Autodesk Inventor part; units mm, degrees
ref_plane "YZ Plane" through (0, 0, 0) normal (1, 0, 0) x (0, 1, 0)
ref_plane "XZ Plane" through (0, 0, 0) normal (0, 1, 0) x (-1, 0, 0)
ref_plane "XY Plane" through (0, 0, 0) normal (0, 0, 1) x (1, 0, 0)
sketch "Sketch1" plane through (0, 0, 0) normal (0, 1, 0) x (-1, 0, 0)
  line L0 (0, 0) -> (-50, 0)
  line L1 (-50, 0) -> (-50, -50)
  line L2 (-50, -50) -> (0, -50)
  line L3 (0, -50) -> (0, 0)
  line L4 (-5, -5) -> (-45, -5)
  line L5 (-45, -5) -> (-45, -45)
  line L6 (-45, -45) -> (-5, -45)
  line L7 (-5, -45) -> (-5, -5)
  dimension "d0" = 50
  dimension "d1" = 50
  dimension "d2" = 5
extrude "Extrusion1" add sketch "Sketch1" along normal blind 5
sketch "Sketch2" plane through (0, 0, 0) normal (0, 0, 1) x (1, 0, 0)
  line L0 (0, 5) -> (50, 5)
  line L1 (13, 5) -> (37, 5)
  line L2 (37, 5) -> (37, 2.5)
  line L3 (37, 2.5) -> (13, 2.5)
  line L4 (13, 2.5) -> (13, 5)
  line L5 (0, 0) -> (50, 0)
  line L6 (0, 0) -> (0, 5)
  dimension "d5" = 24
  dimension "d6" = 2.5
  dimension "d7" = 13
extrude "Extrusion2" cut sketch "Sketch2" against normal through all
sketch "Sketch3" plane through (0, 0, 0) normal (0, 0, 1) x (1, 0, 0)
  line L0 (13, 2.5) -> (13, 5)
  line L1 (13, 5) -> (13, 15)
  line L2 (13, 5) -> (0, 5)
  line L3 (13, 15) -> (0, 5)
  line L4 (37, 5) -> (37, 2.5)
  line L5 (37, 5) -> (37, 15)
  line L6 (50, 5) -> (37, 5)
  line L7 (37, 15) -> (50, 5)
  point P0 (0, 0)
  dimension "d10" = 10
  dimension "d11" = 10
extrude "Extrusion3" add sketch "Sketch3" against normal blind 5
sketch "Sketch4" plane through (50, 0, -50) normal (0, 0, -1) x (-1, 0, 0)
  line L0 (50, 5) -> (37, 15)
  line L1 (37, 15) -> (37, 2.5)
  line L2 (13, 15) -> (0, 5)
  line L3 (13, 2.5) -> (13, 15)
  line L4 (0, 5) -> (13, 15)
  line L5 (13, 5) -> (5, 5)
  line L6 (13, 15) -> (13, 5)
  line L7 (0, 5) -> (13, 5)
  line L8 (13, 5) -> (0, 5)
  line L9 (50, 5) -> (45, 5)
  line L10 (50, 5) -> (37, 15)
  line L11 (45, 5) -> (37, 5)
  line L12 (37, 15) -> (37, 5)
  line L13 (37, 5) -> (50, 5)
  point P0 (50, 0)
extrude "Extrusion4" add sketch "Sketch4" against normal blind 5
sketch "Sketch5" plane through (50, 0, -50) normal (0, 0, -1) x (-1, 0, 0)
  circle A0 centre (39.5, 9) radius 0.5
  circle A1 centre (10.5, 9) radius 0.5
  line L0 (37, 2.5) -> (13, 2.5)
  line L1 (37, 15) -> (37, 2.5)
  line L2 (13, 2.5) -> (13, 15)
  point P0 (50, 0)
  dimension "d16" = 6.5
  dimension "d17" = 6.5
  dimension "d18" = 1
  dimension "d19" = 1
  dimension "d20" = 2.5
  dimension "d21" = 2.5
sketch "Sketch6" plane through (50, 0, -50) normal (0, 0, -1) x (-1, 0, 0)
  point P0 (50, 0)
extrude "Extrusion5" cut sketch "Sketch5" against normal through all
properties part number "MotorMountForPrograming"
Work out the finished part from the listing and answer in its coordinate system (mm). A direction names the side the tool comes from. Give positions to 0.01 mm unless a question says otherwise; leave off trailing zeros. Write each loop counter-clockwise with the first axis right and the second up, starting at its lowest first coordinate (ties: lowest second). Pieces come first, ordered by that corner, then holes. Notation, with made-up numbers: M 67,-37.75 L 76,-37.75 A16 ccw 76,-22.75 Z; hole C 73.25,48 d5. An arc over 180 degrees is marked long. Answer as CSV lines item,"result".
Q1. Find the intervals of material crossed by probe 1 along X at (y, z) = (5, -4); probe 2 along Z at (x, y) = (7, 2.25); probe 3 along Y at (x, z) = (19, -3.5), in increasing order. Write a range as [from, to].
A:
probe 1,"x = [0, 13], [37, 50]"
probe 2,"z = [-50, -45], [-5, 0]"
probe 3,"y = [0, 2.5]"
Q2. A tool of negligible diameter and unlimited length cuts with its end or side. For faces 1 (the flat face through (45, 2, -25)), 2 (the flat face through (25, 2.5, -2)), 3 (the flat face through (48, 5, -25)), from which of +Z, -Z, +X, -X, +Y, -Y can it reach the whole face along a straight path? Write none if from no direction.
A:
face 1,"+Y, -Y"
face 2,"+Z, -Z, +Y"
face 3,"+X, -X, +Y"
Q3. A cutting plane is placed at C-C on x = 36. Write down the section's boundary in (y, z).
A:
outline,"M 0,-50 L 2.5,-50 L 2.5,-45 L 0,-45 Z; M 0,-5 L 2.5,-5 L 2.5,0 L 0,0 Z"
Q4. A cutting plane is placed at D-D on z = -33. Write down the section's boundary in (x, y), plus the area to 3 significant figures.
A:
outline,"M 0,0 L 5,0 L 5,5 L 0,5 Z; M 45,0 L 50,0 L 50,5 L 45,5 Z"
area,"50.0 mm²"
Q5. Given P1, Ø5.5, axis at y = 8, z = -1.5, coming from the +X side (3 decimals); P2, Ø2.5, axis at y = 7.5, z = -47, coming from the +X side (3 decimals); P3, Ø5.5, axis at x = 22.5, z = -3.5, coming from the +Y side, each flat-ended and moving along its own axis, determine where each tip first touches the part or whether it passes through.
A:
P1,"stops at x = 49.675"
P2,"stops at x = 48.375"
P3,"stops at y = 2.5"
Q6. A cutting plane is placed at B-B on z = -3. Write down the section's boundary in (x, y).
A:
outline,"M 0,0 L 50,0 L 50,5 L 37,15 L 37,2.5 L 13,2.5 L 13,15 L 0,5 Z; hole C 10.5,9 d1; hole C 39.5,9 d1"
Q7. A cutting plane is placed at A-A on y = 6.5. Write down the section's boundary in (x, z).
A:
outline,"M 1.95,-50 L 13,-50 L 13,-45 L 1.95,-45 Z; M 1.95,-5 L 13,-5 L 13,0 L 1.95,0 Z; M 37,-50 L 48.05,-50 L 48.05,-45 L 37,-45 Z; M 37,-5 L 48.05,-5 L 48.05,0 L 37,0 Z"
Q8. The mould has two halves that part along X. Classify faces 4 (the flat face through (3, 5, -25)), 5 (the flat face through (0, 2, -25)), 6 (the flat face through (25, 2.5, -47)), 7 (the flat face through (25, 2, -5)): +X half, -X half, draft (parallel to the pull), parting line (faces both ways), or undercut.
A:
face 4,"draft"
face 5,"-X half"
face 6,"undercut"
face 7,"undercut"
